Autodesk Fusion 360 part; units mm, degrees
sketch "Sketch1" plane through (0, 0, 0) normal (0, 1, 0) x (1, 0, 0)
  line L0 (0, 0) -> (-1.6, 0)
  line L1 (-1.6, 0) -> (-1.6, 31)
  line L2 (-1.6, 31) -> (0, 31)
  line L3 (0, 31) -> (0, 0)
  line L4 (7.5, 0) -> (0, 0)
  line L5 (0, 0) -> (0, 1.6)
  line L6 (0, 1.6) -> (7.5, 1.6)
  line L7 (7.5, 1.6) -> (7.5, 0)
  line L8 (-1.6, 31) -> (-31.6, 31)
  line L9 (-31.6, 31) -> (-31.6, 29.4)
  line L10 (-31.6, 29.4) -> (-1.6, 29.4)
  line L11 (-1.6, 29.4) -> (-1.6, 31)
  line L12 (-31.6, 31) -> (-33.2, 31)
  line L13 (-33.2, 31) -> (-33.2, 0)
  line L14 (-33.2, 0) -> (-31.6, 0)
  line L15 (-31.6, 0) -> (-31.6, 31)
  line L16 (-40.7, 1.6) -> (-33.2, 1.6)
  line L17 (-33.2, 1.6) -> (-33.2, 0)
  line L18 (-33.2, 0) -> (-40.7, 0)
  line L19 (-40.7, 0) -> (-40.7, 1.6)
  dimension "d2" = 1.6
  dimension "d3" = 7.5
  dimension "d4" = 1.6
  dimension "d5" = 1.6
  dimension "d6" = 1.6
  dimension "d7" = 30
  dimension "d16" = 29.4
extrude "Extrude1" add sketch "Sketch1" along normal blind 10
hole "Hole1" at (3.75, 5, -1.6) direction (0, 0, 1) diameter 3.5 depth 4 tip angle 118
hole "Hole2" at (-36.95, 5, -1.6) direction (0, 0, 1) diameter 3.5 depth 4 tip angle 118
fillet "Fillet1" radius 6.5 2 edges at (-1.6, 5, -29.4) (-31.6, 5, -29.4)
fillet "Fillet2" radius 8.5 2 edges at (0, 5, -31) (-33.2, 5, -31)
equation "d2 = d4"
equation "d5 = d4"
equation "d6 = d4"
Verification items for the finished model (mm, model axes). A direction names the side the tool comes from. Coordinates: 2 decimals unless noted, no trailing zeros. Loops run counter-clockwise (first coordinate to the right, second up) from the corner with the lowest first, then second, coordinate; pieces in that order, holes last. Notation, with made-up numbers: (72.5, 82.5) -> (108.5, 82.5) arc R21 cw to (108.5, 118.5) -> close; hole circle Ø7 at (-35, 62.25). An arc over 180 degrees is marked (long way). Answer in a Markdown table with one row per item.
1) Depth check by flat-ended pin: P1, Ø1, axis at x = -5, y = 5, coming from the -Z side; P2, Ø4, axis at x = -37, y = 5.5, coming from the -Z side; P3, Ø3, axis at x = 3.75, y = 5, coming from the +Z side; P4, Ø4, axis at y = 2, z = -5.5, coming from the -X side. Enter the tip coordinate at first touch or a pass-through.
The answers:
| item | result |
|---|---|
| P1 | stops at z = -30.45 |
| P2 | stops at z = -1.6 |
| P3 | passes through |
| P4 | stops at x = -33.2 |
2) Section check A-A (y = 5). Record the cut outline in (x, z), and give its area (3 significant figures).
The answers:
| item | result |
|---|---|
| outline | (-40.7, -1.6) -> (-38.7, -1.6) -> (-38.7, 0) -> (-40.7, 0) -> close; (-35.2, -1.6) -> (-33.2, -1.6) -> (-33.2, -22.5) arc R8.5 ccw to (-24.7, -31) -> (-8.5, -31) arc R8.5 ccw to (0, -22.5) -> (0, -1.6) -> (2, -1.6) -> (2, 0) -> (-1.6, 0) -> (-1.6, -22.9) arc R6.5 cw to (-8.1, -29.4) -> (-25.1, -29.4) arc R6.5 cw to (-31.6, -22.9) -> (-31.6, 0) -> (-35.2, 0) -> close; (5.5, -1.6) -> (7.5, -1.6) -> (7.5, 0) -> (5.5, 0) -> close |
| area | 147 mm2 |
3) Access from +Z, -Z, +X, -X, +Y, -Y to the whole of each face (thin tool, end or side, straight path). Record for faces 5 (the face through (-33.2, 5, -12)), 6 (the face through (-3.454, 5.07, -27.445)), 7 (the face through (2, 4, -1.6)).
The answers:
| item | result |
|---|---|
| face 5 | -Z, -X, +Y, -Y |
| face 6 | +Z, +Y, -Y |
| face 7 | -Z, +X, +Y, -Y |
4) Section check C-C (x = -36.95). Record the cut outline in (y, z).
The answers:
| item | result |
|---|---|
| outline | (0, -1.6) -> (3.25, -1.6) -> (3.25, 0) -> (0, 0) -> close; (6.75, -1.6) -> (10, -1.6) -> (10, 0) -> (6.75, 0) -> close |
5) Section check B-B (z = -2.5). Record the cut outline in (x, y), and give its area (3 significant figures).
The answers:
| item | result |
|---|---|
| outline | (-33.2, 0) -> (-31.6, 0) -> (-31.6, 10) -> (-33.2, 10) -> close; (-1.6, 0) -> (0, 0) -> (0, 10) -> (-1.6, 10) -> close |
| area | 32.0 mm2 |
6) Scan lines: line 1 along X through (y, z) = (5, -0.85); line 2 along Y through (x, z) = (3.75, -1.05); line 3 along X through (y, z) = (1.75, -4). Record each from-to range of solid material in increasing order. Write a range as from..to.
The answers:
| item | result |
|---|---|
| line 1 | x = -40.7..-38.7, -35.2..-31.6, -1.6..2, 5.5..7.5 |
| line 2 | y = 0..3.25, 6.75..10 |
| line 3 | x = -33.2..-31.6, -1.6..0 |
7) Section check D-D (y = 2.5). Record the cut outline in (x, z), and give its area (3 significant figures).
The answers:
| item | result |
|---|---|
| outline | (-40.7, -1.6) -> (-33.2, -1.6) -> (-33.2, -22.5) arc R8.5 ccw to (-24.7, -31) -> (-8.5, -31) arc R8.5 ccw to (0, -22.5) -> (0, -1.6) -> (7.5, -1.6) -> (7.5, 0) -> (-1.6, 0) -> (-1.6, -22.9) arc R6.5 cw to (-8.1, -29.4) -> (-25.1, -29.4) arc R6.5 cw to (-31.6, -22.9) -> (-31.6, 0) -> (-40.7, 0) -> close |
| area | 158 mm2 |
8) Draft check along X on faces 1 (the face through (-17, 5, -31)), 2 (the face through (-17, 5, -29.4)), 3 (the face through (7.5, 5, -1)), 4 (the face through (-31.6, 5, -11)). Enter one of: released by +X, released by -X, zero draft, split by the parting line, or undercut.
The answers:
| item | result |
|---|---|
| face 1 | zero draft |
| face 2 | undercut |
| face 3 | released by +X |
| face 4 | undercut |
